Source: three-view drawing plus pictorial views. Frame: mm from the lowest corner of the part. A direction names the side the tool comes from. Round coordinates to 2 decimals unless told otherwise and drop trailing zeros. Write each loop counter-clockwise with the first axis right and the second up, starting at its lowest first coordinate (ties: lowest second). Pieces come first, ordered by that corner, then holes. Notation, with made-up numbers: M 43,-35 L 58,-35 A26 ccw 58,-8 Z; hole C 20,-20 d9. An arc over 180 degrees is marked long. Put each result on its own line as item: value. Start each with the question number.
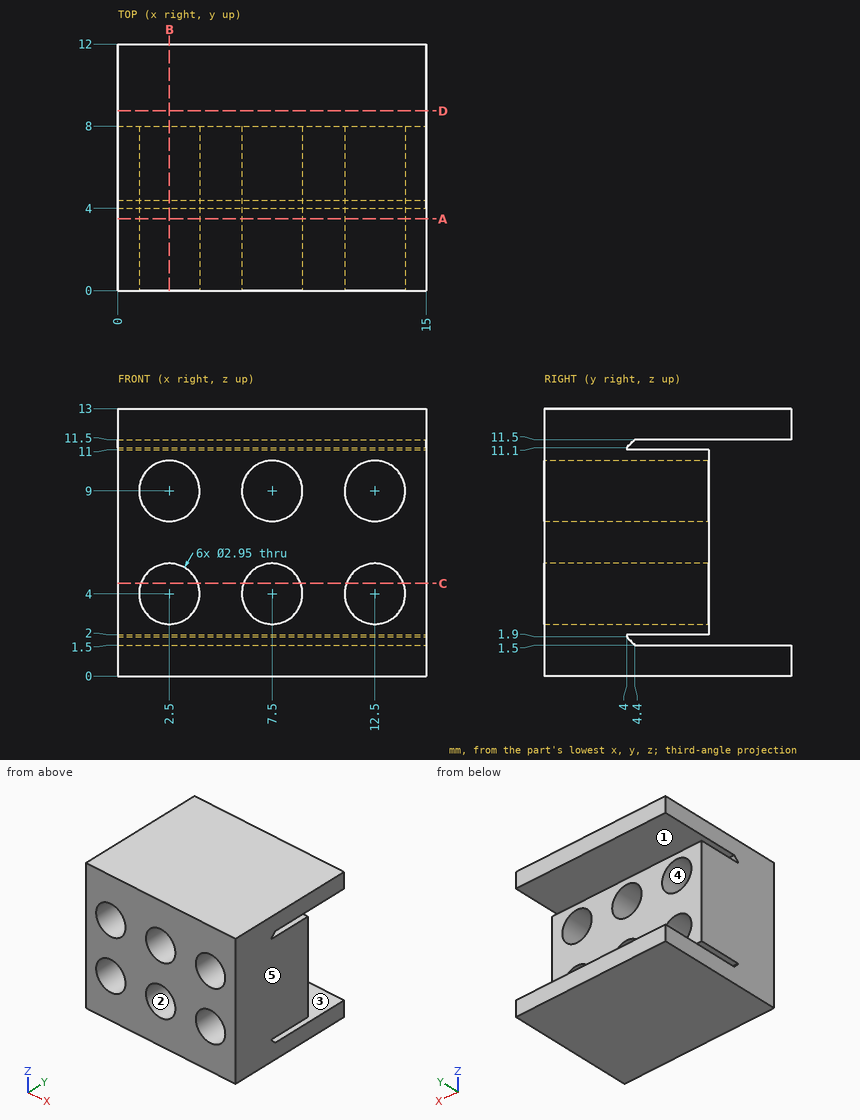
(1) Section query B-B (x = 2.5). Return loops of the section in (y, z) (3 decimals), and give its area (3 significant figures).
(2) Access query for the marked faces 1 and 2. Directions: +Z, -Z, +X, -X, +Y, -Y. A direction counts if a zero-diameter tool reaches every point of the face in a straight line with its end or side. Return the directions, or none.
(3) Section query A-A (y = 3.5). Return loops of the section in (x, z) (3 decimals).
(4) Section query D-D (y = 8.75). Return loops of the section in (x, z), and give its area (3 significant figures).
(5) Ray query, line 1 along X through (y, z) = (6.25, 9) (3 decimals); line 2 along Z through (x, y) = (4.5, 6.5); line 3 along Z through (x, y) = (9, 11.5). Return the intervals inside material, ascending.
(6) Section query C-C (z = 4.5). Return loops of the section in (x, y).
(7) Pull-direction query (X, two-part tool) for the marked faces 3, 4 and 5; classes: +X half, -X half, draft (parallel to the pull), parting line (faces both ways), or undercut.
(8) Contact query for flat-ended pins moving along their axis: P1, Ø1.8, axis at x = 7.5, z = 4, coming from the -Y side; P2, Ø4, axis at x = 7.5, z = 9, coming from the +Y side. Output: stop coordinate, or through.
Entries:
1. outline: M 0,0 L 12,0 L 12,1.5 L 4.4,1.5 L 4,1.9 L 4,2 L 8,2 L 8,2.525 L 0,2.525 Z; M 0,5.475 L 8,5.475 L 8,7.525 L 0,7.525 Z; M 0,10.475 L 8,10.475 L 8,11 L 4,11 L 4,11.1 L 4.4,11.5 L 12,11.5 L 12,13 L 0,13 Z
1. area: 65.0 mm2
2. face 1: +X, -X, +Y
2. face 2: +Y, -Y
3. outline: M 0,0 L 15,0 L 15,13 L 0,13 Z; hole C 2.5,4 d2.95; hole C 2.5,9 d2.95; hole C 7.5,4 d2.95; hole C 7.5,9 d2.95; hole C 12.5,4 d2.95; hole C 12.5,9 d2.95
4. outline: M 0,0 L 15,0 L 15,1.5 L 0,1.5 Z; M 0,11.5 L 15,11.5 L 15,13 L 0,13 Z
4. area: 45.0 mm2
5. line 1: 0 to 1.025, 3.975 to 6.025, 8.975 to 11.025, 13.975 to 15
5. line 2: 0 to 1.5, 2 to 11, 11.5 to 13
5. line 3: 0 to 1.5, 11.5 to 13
6. outline: M 0,0 L 1.11,0 L 1.11,8 L 0,8 Z; M 3.89,0 L 6.11,0 L 6.11,8 L 3.89,8 Z; M 8.89,0 L 11.11,0 L 11.11,8 L 8.89,8 Z; M 13.89,0 L 15,0 L 15,8 L 13.89,8 Z
7. face 3: draft
7. face 4: undercut
7. face 5: +X half
8. P1: through
8. P2: y = 8
